Check sheet for the modelled part. Datum: model origin and axes. Units: mm. Face numbers are marked on the shaded views. A direction names the side the tool comes from. Round coordinates to 2 decimals unless told otherwise and drop trailing zeros. Order: outer loops, then holes, each group sorted by start corner. A loop starts at its lowest first (then second) coordinate and runs counter-clockwise, first axis right, second up.
(1) Sectioned sample at A-A, the plane x = -13. Enter the section's corners in (y, z), and give its area (3 significant figures).
(2) Sectioned sample at D-D, the plane y = -5. Enter the section's corners in (x, z), and give its area (3 significant figures).
(3) Tool access check on the marked faces 1, 2, 3, 4 and 5. Record the directions out of +Z, -Z, +X, -X, +Y, -Y that give a thin tool (end or side, any length) a straight path to the whole face; none if there is none.
(4) Sectioned sample at C-C, the plane z = 1. Count the separate pieces of the cut face and the enclosed holes in it, and give its area (3 significant figures).
(5) Depth check by flat-ended pin: pin 1 (4 mm diameter, centred on y = -16.51, z = 0, fed in from -X); pin 2 (10 mm diameter, centred on x = -5, y = -5, fed in from +Z); pin 3 (5 mm diameter, centred on x = 8, z = 7, fed in from -Y); pin 4 (2 mm diameter, centred on y = -2, z = 0.5, fed in from +X). Enter the tip coordinate at first touch or a pass-through.
(6) Thickness scan on probe 1 along Y at (x, z) = (11, 0) (3 decimals); probe 2 along X at (y, z) = (-28.5, -6) (1 decimal); probe 3 along Z at (x, y) = (-1, -1.5). Record the ranges inside material, lowest first.
(7) Mould release check, pull along X, two halves, no side actions. Record for the marked faces 6, 7 and 8: released by +X, released by -X, zero draft, split by the parting line, or undercut.
(8) Sectioned sample at B-B, the plane y = -16.51. Enter the section's corners in (x, z) (1 decimal), and give its area (3 significant figures).
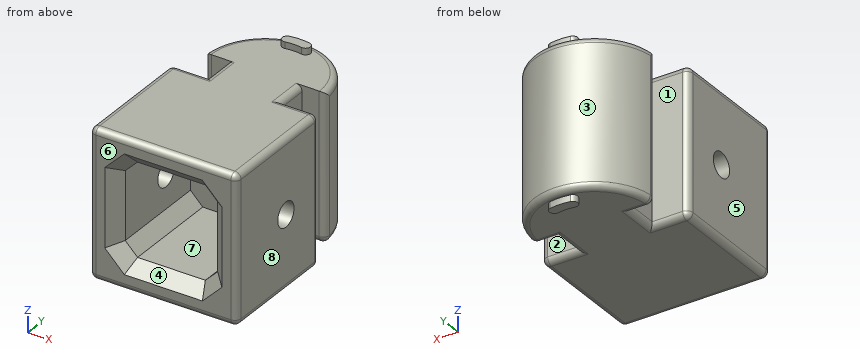
```python
from build123d import *

# Parameters (mm, degrees)
MAIN_BODY_EXTRUDE_DEPTH   = 15.1765
SLOT_EXTRUDE_DEPTH        = 16.51
SKETCH2_W                 = 19.05
SKETCH2_H                 = 19.05
FOOT_CONNECTION_CUT_DEPTH = 22.86
SKETCH4_R                 = 2.54
PINHOLE_CUT_DEPTH         = 25.4
FILLET1_R                 = 1.27
CHAMFER2_SIZE             = 2.54
CHAMFER1_SIZE             = 2.54


with BuildPart() as part:
    # Sketch1 → Main Body Extrude (new body, symmetric)
    with BuildSketch(Plane.XY):
        with BuildLine():
            Line((-12.446, 0), (12.446, 0))
            ThreePointArc((12.446, 0), (0, 12.446), (-12.446, 0))
        make_face()
        with BuildLine():
            ThreePointArc((2.100384615, 10.71813736), (0, 10.922), (-2.100384615, 10.71813736))
            ThreePointArc((-2.100384615, 10.71813736), (-2.902036033, 9.525716711), (-1.709615385, 8.724065293))
            ThreePointArc((-1.709615385, 8.724065293), (0, 8.89), (1.709615385, 8.724065293))
            ThreePointArc((1.709615385, 8.724065293), (2.902036033, 9.525716711), (2.100384615, 10.71813736))
        make_face(mode=Mode.SUBTRACT)
        Polygon((-7.62, 0), (7.62, 0), (7.62, -6.35), (15.1765, -6.35), (15.1765, -31.75), (-15.1765, -31.75), (-15.1765, -6.35), (-7.62, -6.35), align=None)
    extrude(amount=MAIN_BODY_EXTRUDE_DEPTH, both=True)

    # Sketch1_4 → Slot Extrude (add, symmetric)
    with BuildSketch(Plane.XY):
        with BuildLine():
            ThreePointArc((-2.100384615, 10.71813736), (-2.902036033, 9.525716711), (-1.709615385, 8.724065293))
            ThreePointArc((-1.709615385, 8.724065293), (0, 8.89), (1.709615385, 8.724065293))
            ThreePointArc((1.709615385, 8.724065293), (2.902036033, 9.525716711), (2.100384615, 10.71813736))
            ThreePointArc((2.100384615, 10.71813736), (0, 10.922), (-2.100384615, 10.71813736))
        make_face()
    extrude(amount=SLOT_EXTRUDE_DEPTH, both=True)

    # Sketch2 → Foot Connection Cut (cut)
    with BuildSketch(Plane.XZ.offset(31.75)):
        Rectangle(SKETCH2_W, SKETCH2_H)
    extrude(amount=-FOOT_CONNECTION_CUT_DEPTH, mode=Mode.SUBTRACT)

    # Sketch4 → Pinhole Cut (cut, symmetric)
    with BuildSketch(Plane(origin=(-9.525, 0, 0), x_dir=(0, 0, -1), z_dir=(1, 0, 0))):
        with Locations((0, -16.51)):
            Circle(SKETCH4_R)
    extrude(amount=PINHOLE_CUT_DEPTH, both=True, mode=Mode.SUBTRACT)

    # Fillet1
    fillet1_edges = [part.edges().sort_by_distance(p)[0] for p in [
        (15.1765, -19.05, 15.1765),
        (-11.39825, -6.35, -15.1765),
        (-7.62, -3.175, -15.1765),
        (7.62, -3.175, -15.1765),
        (11.39825, -6.35, -15.1765),
        (15.1765, -19.05, -15.1765),
        (0, -31.75, -15.1765),
        (11.39825, -6.35, 15.1765),
        (-15.1765, -31.75, 0),
        (-15.1765, -6.35, 0),
        (15.1765, -6.35, 0),
        (15.1765, -31.75, 0),
        (7.62, -3.175, 15.1765),
        (-7.62, -3.175, 15.1765),
        (12.446, 0, 0),
        (-12.446, 0, 0),
        (0, 12.446, 15.1765),
        (0, 12.446, -15.1765),
        (-10.033, 0, -15.1765),
        (10.033, 0, -15.1765),
        (-11.39825, -6.35, 15.1765),
        (-15.1765, -19.05, 15.1765),
        (0, -31.75, 15.1765),
        (-15.1765, -19.05, -15.1765),
    ]]
    fillet(fillet1_edges, radius=FILLET1_R)

    # Chamfer2
    chamfer2_edges = [part.edges().sort_by_distance(p)[0] for p in [
        (9.525, -20.32, 9.525),
        (9.525, -20.32, -9.525),
        (-9.525, -20.32, -9.525),
        (-9.525, -20.32, 9.525),
    ]]
    chamfer(chamfer2_edges, length=CHAMFER2_SIZE)

    # Chamfer1
    chamfer1_edges = [part.edges().sort_by_distance(p)[0] for p in [
        (0, -31.75, -9.525),
        (-9.525, -31.75, 0),
        (0, -31.75, 9.525),
        (9.525, -31.75, 0),
        (-8.255, -31.75, -8.255),
        (-8.255, -31.75, 8.255),
        (8.255, -31.75, -8.255),
        (8.255, -31.75, 8.255),
    ]]
    chamfer(chamfer1_edges, length=CHAMFER1_SIZE)


solid = part.part
```
Derived:
1. outline: (-31.75, -13.91) arc R1.27 ccw to (-30.48, -15.18) - (-7.62, -15.18) arc R1.27 ccw to (-6.35, -13.91) - (-6.35, 13.91) arc R1.27 ccw to (-7.62, 15.18) - (-30.48, 15.18) arc R1.27 ccw to (-31.75, 13.91) - close; hole circle Ø5.08 at (-16.51, 0)
1. area: 749 mm2
2. outline: (-7.62, -13.91) arc R1.27 ccw to (-6.35, -15.18) - (6.35, -15.18) arc R1.27 ccw to (7.62, -13.91) - (7.62, 13.91) arc R1.27 ccw to (6.35, 15.18) - (-6.35, 15.18) arc R1.27 ccw to (-7.62, 13.91) - close
2. area: 461 mm2
3. face 1: +Z, -Z, -X
3. face 2: +Z, -Z, +X
3. face 3: +Z, -Z, +Y
3. face 4: -Y
3. face 5: +Z, -Z, -X, +Y, -Y
4. separate pieces: 3
4. enclosed holes: 0
4. area: 614 mm2
5. pin 1: passes through
5. pin 2: stops at z = 15.18
5. pin 3: stops at y = -30.64
5. pin 4: stops at x = 7.62
6. probe 1: y = -30.685 to -19.05, -13.97 to -6.35, 0 to 5.823
6. probe 2: x = -15.2 to -9.5, 9.5 to 15.2
6. probe 3: z = -15.18 to 15.18
7. face 6: zero draft
7. face 7: undercut
7. face 8: released by +X
8. outline: (-15.2, -13.9) arc R1.3 ccw to (-13.9, -15.2) - (13.9, -15.2) arc R1.3 ccw to (15.2, -13.9) - (15.2, -2.5) - (9.5, -2.5) - (9.5, -7) - (7, -9.5) - (-7, -9.5) - (-9.5, -7) - (-9.5, -2.5) - (-15.2, -2.5) - close; (-15.2, 2.5) - (-9.5, 2.5) - (-9.5, 7) - (-7, 9.5) - (7, 9.5) - (9.5, 7) - (9.5, 2.5) - (15.2, 2.5) - (15.2, 13.9) arc R1.3 ccw to (13.9, 15.2) - (-13.9, 15.2) arc R1.3 ccw to (-15.2, 13.9) - close
8. area: 513 mm2
